Check sheet for the modelled part. Datum: model origin and axes. Units: mm. A direction names the side the tool comes from. Coordinates: 2 decimals unless noted, no trailing zeros. Loops run counter-clockwise (first coordinate to the right, second up) from the corner with the lowest first, then second, coordinate; pieces in that order, holes last. Notation, with made-up numbers: M -15,56 L 29,56 A21 cw 29,82 Z; hole C 18,20.5 d10. An arc over 180 degrees is marked long. Return JSON: item names as keys, results as strings.
Autodesk Inventor part; units mm, degrees
ref_plane "YZ Plane" through (0, 0, 0) normal (1, 0, 0) x (0, 1, 0)
ref_plane "XZ Plane" through (0, 0, 0) normal (0, 1, 0) x (-1, 0, 0)
ref_plane "XY Plane" through (0, 0, 0) normal (0, 0, 1) x (1, 0, 0)
sketch "Sketch1" plane through (0, 0, 0) normal (0, 0, 1) x (1, 0, 0)
  circle A0 centre (0, 0) radius 29.5
  circle A1 centre (0, 0) radius 16 construction
  circle A2 centre (0, 0) radius 12.5 construction
  circle A3 centre (0, 0) radius 8.5
  line L0 (0, 0) -> (17.0589, 17.0589) construction
  line L1 (-45.7937, 0) -> (68.262, 0)
  line L2 (0, 0) -> (-17.0589, 17.0589) construction
  line L3 (0, 0) -> (-17.0589, -17.0589) construction
  line L4 (0, 0) -> (17.0589, -17.0589) construction
  line L5 (0, 0) -> (51.9684, 0) construction
  line L6 (0, 0) -> (-25.9842, 45.0059) construction
  line L7 (0, 0) -> (-25.9842, -45.0059) construction
  circle A4 centre (0, 0) radius 3 construction
  circle A5 centre (0, 0) radius 2 construction
  point P0 (8.5, 0)
  point P1 (-4.25, 7.3612)
  point P2 (-4.25, -7.3612)
  point P3 (8.8388, 8.8388)
  point P4 (-8.8388, -8.8388)
  point P5 (-8.8388, 8.8388)
  point P6 (8.8388, -8.8388)
  point P7 (16, 0)
  point P8 (-8, -13.8564)
  point P9 (-8, 13.8564)
  dimension "d0" = 59
  dimension "d1" = 32
  dimension "d2" = 25
  dimension "d3" = 17
  dimension "d4" = 45
  dimension "d8" = 360
  dimension "d12" = 360
  dimension "d14" = 6
  dimension "d15" = 4
sketch "Sketch2" plane through (0, 0, 0) normal (0, 0, 1) x (1, 0, 0)
  circle A0 centre (0, 0) radius 29.5
extrude "Extrusion1" add sketch "Sketch2" along normal mid plane 42.5
sketch "Sketch3" plane through (0, 0, 21.25) normal (0, 0, 1) x (1, 0, 0)
  circle A0 centre (0, 0) radius 2
  circle A1 centre (0, 0) radius 29.5
extrude "Extrusion2" cut sketch "Sketch3" against normal blind 6
sketch "Sketch4" plane through (0, 0, -21.25) normal (0, 0, -1) x (-1, 0, 0)
  circle A0 centre (0, 0) radius 3
  circle A1 centre (0, 0) radius 29.5
extrude "Extrusion3" cut sketch "Sketch4" against normal blind 3
sketch "Sketch5" plane through (0, 0, 15.25) normal (0, 0, 1) x (1, 0, 0)
  circle A0 centre (0, 0) radius 8.5
  circle A1 centre (0, 0) radius 12.5
  point P0 (-4.25, 7.3612)
  point P1 (8.5, 0)
  point P2 (-4.25, -7.3612)
  dimension "d29" = 25
hole "Hole1" at (-4.25, 7.3612, 15.25) at (8.5, 0, 15.25) at (-4.25, -7.3612, 15.25) direction (0, 0, -1) diameter 3 depth 5 tip angle 118
chamfer "Chamfer1" distance 8.8 distance2 17 1 edges at (-29.5, 0, 15.25) measured on face at (29.4043, -2.3738, -7.0833)
sketch "Sketch6" plane through (0, 0, -21.25) normal (0, 0, -1) x (-1, 0, 0)
  circle A0 centre (0, 0) radius 3
extrude "Magnet" add sketch "Sketch6" along normal blind 2
chamfer "Chamfer2" distance 4.5 distance2 7.5 1 edges at (-29.5, 0, -18.25) measured on face at (29.118, -4.7321, -10.0167)
sketch "Sketch7" plane through (0, 0, -18.25) normal (0, 0, -1) x (-1, 0, 0)
  circle A0 centre (0, 0) radius 8.5
  circle A1 centre (0, 0) radius 12.5
  point P0 (8.8388, 8.8388)
  point P1 (-8.8388, 8.8388)
  point P2 (-8.8388, -8.8388)
  point P3 (8.8388, -8.8388)
  point P4 (8, 13.8564)
  point P5 (8, -13.8564)
  point P6 (-16, 0)
hole "Hole2" at (8.8388, 8.8388, -18.25) at (-8.8388, 8.8388, -18.25) at (-8.8388, -8.8388, -18.25) at (8.8388, -8.8388, -18.25) direction (0, 0, 1) diameter 3 depth 4 tip angle 118
hole "Hole3" at (-8, 13.8564, -18.25) at (16, 0, -18.25) at (-8, -13.8564, -18.25) direction (0, 0, 1) diameter 2.5 depth 3 tip angle 118
sketch "Sketch8" plane through (0, 0, -23.25) normal (0, 0, -1) x (-1, 0, 0)
  line L0 (-1.6203, 1.7761) -> (1.6105, 1.7761) construction
  line L1 (1.6105, 1.7761) -> (1.6105, -1.2719) construction
  line L2 (1.6105, -1.2719) -> (-1.6203, -1.2719) construction
  line L3 (-1.6203, -1.2719) -> (-1.6203, 1.7761) construction
  line L4 (1.3017, -1.2719) -> (0.8967, -1.2719)
  line L5 (0.8967, -1.2719) -> (0.8967, 1.3537)
  line L6 (0.8967, 1.3537) -> (0.1013, -0.4321)
  line L7 (0.1013, -0.4321) -> (-0.1457, -0.4321)
  line L8 (-0.1457, -0.4321) -> (-0.9336, 1.3537)
  line L9 (-0.9336, 1.3537) -> (-0.9336, -1.2719)
  line L10 (-0.9336, -1.2719) -> (-1.3115, -1.2719)
  line L11 (-1.3115, -1.2719) -> (-1.3115, 1.7761)
  line L12 (-1.3115, 1.7761) -> (-0.7583, 1.7761)
  line L13 (-0.7583, 1.7761) -> (0.0025, 0.0792)
  line L14 (0.0025, 0.0792) -> (0.7386, 1.7761)
  line L15 (0.7386, 1.7761) -> (1.3017, 1.7761)
  line L16 (1.3017, 1.7761) -> (1.3017, -1.2719)
  point P0 (0, 0)
extrude "Extrusion5" cut sketch "Sketch8" against normal blind 0.5
sketch "Sketch9" plane through (0, 0, -18.25) normal (0, 0, -1) x (-1, 0, 0)
  circle A0 centre (-8.8388, 8.8388) radius 1.5
  circle A1 centre (8.8388, 8.8388) radius 1.5
  circle A2 centre (8.8388, -8.8388) radius 1.5
  circle A3 centre (-8.8388, -8.8388) radius 1.5
  circle A4 centre (0, 0) radius 3
  circle A5 centre (0, 0) radius 29.5
  circle A6 centre (-16, 0) radius 1.25
  circle A7 centre (8, 13.8564) radius 1.25
  circle A8 centre (8, -13.8564) radius 1.25
equation "\"d22\" = M3"
equation "\"d27\" = D5_M3"
equation "\"d38\" = M3"
equation "\"M3\" = 3"
equation "\"D5_M3\" = 5"
properties part number "3phaseMotor"
1) Draft check along X on faces 4 (the face through (-5, 0, -18.25)), 5 (the face through (8.269, -0.12, 9.505)), 6 (the face through (28.14, -8.86, -3.79)), 7 (the face through (-9.07, 8.959, -13.505)). Enter one of: +X half, -X half, draft (parallel to the pull), parting line (faces both ways), or undercut.
Answers:
{"face 4": "draft", "face 5": "undercut", "face 6": "parting line", "face 7": "undercut"}
2) Go/stop test with flat-tipped pins: pin 1 Ø1 at (x, y) = (-4, -17) entering from +Z; pin 2 Ø3 at (x, y) = (-8, 13.86) entering from +Z; pin 3 Ø5 at (x, y) = (-4.25, -7.36) entering from -Z. Record where each tip stops, or that it passes through.
Answers:
{"pin 1": "z = 12.94", "pin 2": "z = 14.21", "pin 3": "z = -18.25"}
3) Section check A-A on z = 4. Record the cut outline in (x, y), then the cut area to 3 significant figures.
Answers:
{"outline": "C 0,0 d59", "area": "2,730 mm²"}
4) Section check B-B on z = -20. Record the cut outline in (x, y).
Answers:
{"outline": "C 0,0 d6"}
5) Scan lines: line 1 along Y through (x, z) = (-4.25, 13.65); line 2 along Y through (x, z) = (16, -16.65); line 3 along Z through (x, y) = (4.5, 4.5). Record each from-to range of solid material in increasing order. Write a range as [from, to].
Answers:
{"line 1": "[-15, -8.86], [-5.86, 5.86], [8.86, 15]", "line 2": "[-18.77, -1.25], [1.25, 18.77]", "line 3": "[-18.25, 15.25]"}
6) Set-up check for faces 1 (the face through (14.76, -0.16, -16.73)), 2 (the face through (0, -1, -23.25)), 3 (the face through (-4.32, 8.86, 12.72)): record each of +Z, -Z, +X, -X, +Y, -Y from which the full face is reachable in a straight line by a thin tool's end or side.
Answers:
{"face 1": "-Z", "face 2": "-Z, +X, -X, +Y, -Y", "face 3": "+Z"}
